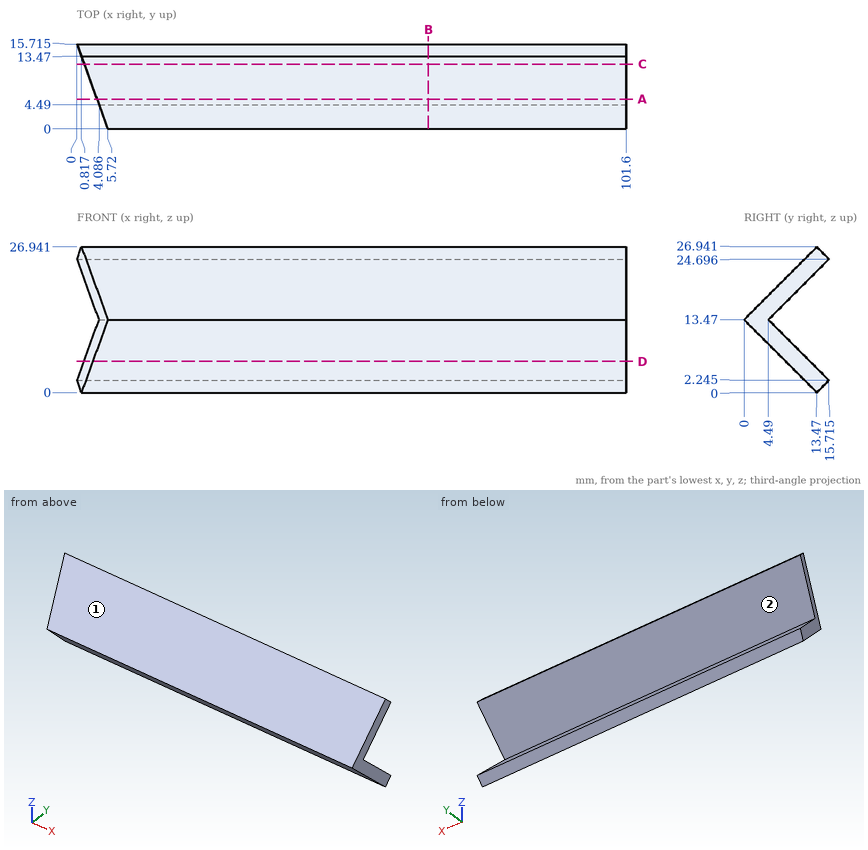
Design review of the part shown in the three views and the two pictorial views. Dimensions are in mm from the part's minimum x, y and z. Round coordinates to 2 decimals unless told otherwise and drop trailing zeros. Loops run counter-clockwise (first coordinate to the right, second up) from the corner with the lowest first, then second, coordinate; pieces in that order, holes last.
1) Consider section C-C on y = 12. State the section outline as (x, z) points.
Values follow:
outline: (1.35, 1.47) - (101.6, 1.47) - (101.6, 5.96) - (1.35, 5.96) - close; (1.35, 20.98) - (101.6, 20.98) - (101.6, 25.47) - (1.35, 25.47) - close
2) Wall thickness on line 1 along Z through (x, y) = (46.5, 6.25); line 2 along Z through (x, y) = (9.5, 12); line 3 along Y through (x, z) = (51.5, 16.5): over which ranges is each line inside the solid? List them lowest first.
Values follow:
line 1: z = 7.22 to 11.71, 15.23 to 19.72
line 2: z = 1.47 to 5.96, 20.98 to 25.47
line 3: y = 3.03 to 7.52
3) Clearance check with flat-ended pins moving along their axes: P1, Ø5, axis at x = 42, y = 5, coming from the -Z side; P2, Ø3, axis at x = 88, y = 2.5, coming from the -Z side; P3, Ø6, axis at x = 60.5, z = 5.5, coming from the +Y side. State where each tip first meets the part, or that it passes through.
Values follow:
P1: stops at z = 5.97
P2: stops at z = 9.47
P3: stops at y = 15.46
4) Consider section D-D on z = 5.75. State the section outline as (x, y) points (1 decimal), then the cut area to 3 significant figures.
Values follow:
outline: (1.3, 12.2) - (2.9, 7.7) - (101.6, 7.7) - (101.6, 12.2) - close
area: 447 mm2
5) Consider section B-B on x = 65. State the section outline as (y, z) points (1 decimal), then the cut area to 3 significant figures.
Values follow:
outline: (0, 13.5) - (13.5, 0) - (15.7, 2.2) - (4.5, 13.5) - (15.7, 24.7) - (13.5, 26.9) - close
area: 111 mm2
6) The part is to be moulded in two halves that separate along Z. For the marked faces 1 and 2, say which applies: pulls with the +Z half, pulls with the -Z half, needs draft (parallel to the pull), parting line crosses it, or undercut.
Values follow:
face 1: pulls with the +Z half
face 2: undercut
7) Consider section A-A on y = 5.5. State the section outline as (x, z) points, then the cut area to 3 significant figures.
Values follow:
outline: (3.72, 7.97) - (101.6, 7.97) - (101.6, 12.46) - (3.72, 12.46) - close; (3.72, 14.48) - (101.6, 14.48) - (101.6, 18.97) - (3.72, 18.97) - close
area: 879 mm2
